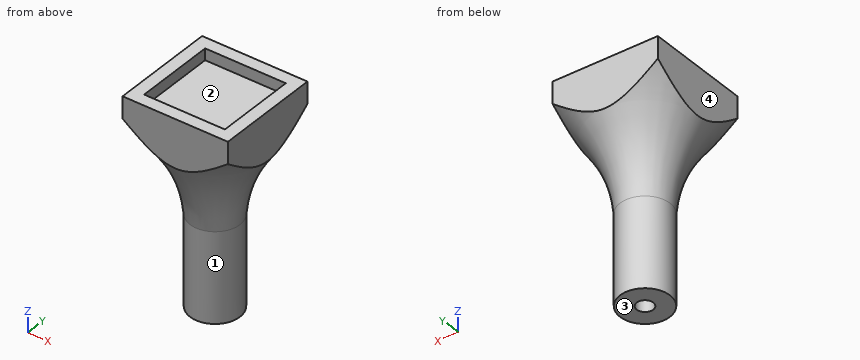
from build123d import *

# Parameters (mm, degrees)
SKETCH1_R           = 6.5
BOSS_EXTRUDE1_DEPTH = 50
SKETCH2_W           = 27.4
SKETCH2_H           = 27.4
BOSS_EXTRUDE2_DEPTH = 5
SKETCH3_W           = 21
SKETCH3_H           = 21
CUT_EXTRUDE1_DEPTH  = 3
SKETCH7_W           = 47.139349652
SKETCH7_H           = 47.139349652
SKETCH7_W_2         = 27.4
SKETCH7_H_2         = 27.4
CUT_EXTRUDE2_DEPTH  = 78
SKETCH8_R           = 2.15
CUT_EXTRUDE3_DEPTH  = 25
CUT_EXTRUDE4_DEPTH  = 3.5
SKETCH10_R          = 2.15
CUT_EXTRUDE5_DEPTH  = 15


with BuildPart() as part:
    # Sketch1 → Boss-Extrude1 (new body)
    with BuildSketch(Plane.XY):
        Circle(SKETCH1_R)
    extrude(amount=BOSS_EXTRUDE1_DEPTH)

    # Sketch2 → Boss-Extrude2 (add)
    with BuildSketch(Plane.XY.offset(50)):
        Rectangle(SKETCH2_W, SKETCH2_H)
    extrude(amount=BOSS_EXTRUDE2_DEPTH)

    # Sketch3 → Cut-Extrude1 (cut)
    with BuildSketch(Plane.XY.offset(55)):
        Rectangle(SKETCH3_W, SKETCH3_H)
    extrude(amount=-CUT_EXTRUDE1_DEPTH, mode=Mode.SUBTRACT)

    # Sketch6 → Revolve1 (revolve)
    with BuildSketch(Plane(origin=(0, 0, 0), x_dir=(0, 0, -1), z_dir=(1, 0, 0))):
        with BuildLine():
            Line((-50, 0), (-50, 20))
            add(Edge.make_bspline(
                [(-50, 20), (-32.330139343, 3.31447133), (-23.53449028, 6.5), (0, 6.5)],
                knots=[0, 0, 0, 0, 1, 1, 1, 1], degree=3))
            Line((0, 6.5), (0, 0))
            Line((0, 0), (-50, 0))
        make_face()
    revolve(axis=Axis((0, 0, 63.541170981), (0, 0, 1)))

    # Sketch7 → Cut-Extrude2 (cut)
    with BuildSketch(Plane.XY.offset(50)):
        Rectangle(SKETCH7_W, SKETCH7_H)
        Rectangle(SKETCH7_W_2, SKETCH7_H_2, mode=Mode.SUBTRACT)
    extrude(amount=-CUT_EXTRUDE2_DEPTH, mode=Mode.SUBTRACT)

    # Sketch8 → Cut-Extrude3 (cut)
    with BuildSketch(Plane(origin=(0, 0, 0), x_dir=(-1, 0, 0), z_dir=(0, 0, -1))):
        Circle(SKETCH8_R)
    extrude(amount=-CUT_EXTRUDE3_DEPTH, mode=Mode.SUBTRACT)

    # Sketch9 → Cut-Extrude4 (cut)
    with BuildSketch(Plane(origin=(0, 0, 25), x_dir=(-1, 0, 0), z_dir=(0, 0, -1))):
        Polygon((4.156921938, 0), (2.078460969, 3.6), (-2.078460969, 3.6), (-4.156921938, 0), (-2.078460969, -3.6), (2.078460969, -3.6), align=None)
    extrude(amount=-CUT_EXTRUDE4_DEPTH, mode=Mode.SUBTRACT)

    # Sketch10 → Cut-Extrude5 (cut)
    with BuildSketch(Plane(origin=(0, 0, 28.5), x_dir=(-1, 0, 0), z_dir=(0, 0, -1))):
        Circle(SKETCH10_R)
    extrude(amount=-CUT_EXTRUDE5_DEPTH, mode=Mode.SUBTRACT)


solid = part.part
Build history of the part. All positions in model axes, mm. Face numbers are marked on the shaded views. Coordinates: 2 decimals unless noted, no trailing zeros. Use CSV: the item, a comma, the result in double quotes. Start each with the question number.
Q1. Pull direction X, two halves, no side cores. Call the marked faces 1, 2, 3 and 4: released by +X, released by -X, zero draft, split by the parting line, or undercut.
Q2. Flat gauge pins, fed straight in: pin 1 Ø3 at (y, z) = (-6.5, 28) entering from -X; pin 2 Ø2 at (x, z) = (-3, 32) entering from -Y; pin 3 Ø1 at (x, z) = (0.5, 26.5) entering from +Y. Where does each tip first touch, or does it go through?
Q3. Drill centre lines: probe 1 along Y at (x, z) = (0, 10.75); probe 2 along Y at (x, z) = (0, 39.75); probe 3 along X at (y, z) = (-1.5, 7.5). Where is each one in solid material? Low to high.
Checked values:
1,face 1,"split by the parting line"
1,face 2,"undercut"
1,face 3,"zero draft"
1,face 4,"released by -X"
2,pin 1,"stops at x = -5.16"
2,pin 2,"stops at y = -8.11"
2,pin 3,"stops at y = 6.95"
3,probe 1,"y = -6.5 to -2.15, 2.15 to 6.5"
3,probe 2,"y = -11.86 to -2.15, 2.15 to 11.86"
3,probe 3,"x = -6.32 to -1.54, 1.54 to 6.32"
